Design review of the part built by this model. Coordinates are the model's own, in mm. Round coordinates to 2 decimals unless told otherwise and drop trailing zeros. Order: outer loops, then holes, each group sorted by start corner. A loop starts at its lowest first (then second) coordinate and runs counter-clockwise, first axis right, second up. Notation, with made-up numbers: (63, 89.5) - (78, 89.5) arc R14 cw to (78, 101.5) - close; hole circle Ø11 at (-22, -28). An arc over 180 degrees is marked (long way). Use CSV: the item, a comma, the result in double quotes. Start each with the question number.
from build123d import *

# Parameters (mm, degrees)
SKETCH_1_R      = 2.5
SKETCH_1_R_2    = 11
SKETCH_1_R_3    = 5
SKETCH_1_R_4    = 1.5
EXTRUDE_1_DEPTH = 2


with BuildPart() as part:
    # 草图1 → 凸台-拉伸1 (new body)
    with BuildSketch(Plane.XY):
        with BuildLine():
            Line((-200.597014925, 350), (59.402985075, 350))
            ThreePointArc((59.402985075, 350), (80.61618851, 341.213203436), (89.402985075, 320))
            Line((89.402985075, 320), (89.402985075, -20))
            ThreePointArc((89.402985075, -20), (80.61618851, -41.213203436), (59.402985075, -50))
            Line((59.402985075, -50), (-200.597014925, -50))
            ThreePointArc((-200.597014925, -50), (-221.810218361, -41.213203436), (-230.597014925, -20))
            Line((-230.597014925, -20), (-230.597014925, 320))
            ThreePointArc((-230.597014925, 320), (-221.810218361, 341.213203436), (-200.597014925, 350))
        make_face()
        with Locations((-190.594777504, 260.002592391)):
            Circle(SKETCH_1_R, mode=Mode.SUBTRACT)
        with Locations((49.405222496, 260.002592391)):
            Circle(SKETCH_1_R, mode=Mode.SUBTRACT)
        with Locations((-140.594777504, -9.997407609)):
            Circle(SKETCH_1_R, mode=Mode.SUBTRACT)
        with Locations((-0.594777504, -9.997407609)):
            Circle(SKETCH_1_R, mode=Mode.SUBTRACT)
        with Locations((-110.597014925, 329)):
            Circle(SKETCH_1_R_2, mode=Mode.SUBTRACT)
        with Locations((-30.597014925, 329)):
            Circle(SKETCH_1_R_2, mode=Mode.SUBTRACT)
        with Locations((-190.597014925, 329)):
            Circle(SKETCH_1_R_2, mode=Mode.SUBTRACT)
        with Locations((49.402985075, 329)):
            Circle(SKETCH_1_R_2, mode=Mode.SUBTRACT)
        with Locations((-210.597014925, 35)):
            Circle(SKETCH_1_R_3, mode=Mode.SUBTRACT)
        with Locations((69.402985075, 35)):
            Circle(SKETCH_1_R_3, mode=Mode.SUBTRACT)
        with Locations((-110.599294274, 247.104711047)):
            Circle(SKETCH_1_R_4, mode=Mode.SUBTRACT)
        with Locations((-110.599294274, 153.604711047)):
            Circle(SKETCH_1_R_4, mode=Mode.SUBTRACT)
        with Locations((3.900705726, 153.604711047)):
            Circle(SKETCH_1_R_4, mode=Mode.SUBTRACT)
        with Locations((3.900705726, 247.104711047)):
            Circle(SKETCH_1_R_4, mode=Mode.SUBTRACT)
        with Locations((-200.598097779, 223.669448039)):
            Circle(SKETCH_1_R_4, mode=Mode.SUBTRACT)
        with Locations((-152.398097779, 223.669448039)):
            Circle(SKETCH_1_R_4, mode=Mode.SUBTRACT)
        with Locations((-200.598097779, 175.469448039)):
            Circle(SKETCH_1_R_4, mode=Mode.SUBTRACT)
        with Locations((-152.398097779, 175.469448039)):
            Circle(SKETCH_1_R_4, mode=Mode.SUBTRACT)
        with Locations((-30.597014925, 280)):
            Circle(SKETCH_1_R_3, mode=Mode.SUBTRACT)
        with Locations((-190.594777504, 280)):
            Circle(SKETCH_1_R_3, mode=Mode.SUBTRACT)
        with Locations((-110.599294274, 280)):
            Circle(SKETCH_1_R_3, mode=Mode.SUBTRACT)
        with Locations((49.405222496, 280)):
            Circle(SKETCH_1_R_3, mode=Mode.SUBTRACT)
    extrude(amount=EXTRUDE_1_DEPTH)


solid = part.part
Q1. Take a section at B-B (y = 35). State the section outline as (x, z) points, plus the area to 3 significant figures.
Q2. For L1, parallel to Y at x = 3, z = 0.55; L2, parallel to X at y = 327.5, z = 0.9; L3, parallel to Y at x = -107.5, z = 0.55, list the stretches that pass through material, from the lowest coordinate up. Write a range as [from, to].
Q3. Take a section at C-C (z = 1.25). Give the number of separate pieces and of enclosed holes in the cut face, plus the area to 3 significant figures.
Q4. Take a section at D-D (y = 329). State the section outline as (x, z) points, plus the area to 3 significant figures.
Q5. The part is to be moulded in two halves that separate along Y. For faces 1 (the cylindrical face through (-191.246, 284.957, 0.986)), 2 (the flat face through (-68, 153, 0)), 3 (the cylindrical face through (80.848, -40.979, 0.986)), say which applies: +Y half, -Y half, draft (parallel to the pull), parting line (faces both ways), or undercut.
Q6. Take a section at A-A (y = 280). State the section outline as (x, z) points.
Findings below:
1,outline,"(-230.6, 0) - (-215.6, 0) - (-215.6, 2) - (-230.6, 2) - close; (-205.6, 0) - (64.4, 0) - (64.4, 2) - (-205.6, 2) - close; (74.4, 0) - (89.4, 0) - (89.4, 2) - (74.4, 2) - close"
1,area,"600 mm^2"
2,L1,"y = [-50, 152.41], [154.8, 245.91], [248.3, 350]"
2,L2,"x = [-229.64, -201.49], [-179.7, -121.49], [-99.7, -41.49], [-19.7, 38.51], [60.3, 88.45]"
2,L3,"y = [-50, 276.08], [283.92, 318.44], [339.56, 350]"
3,separate pieces,"1"
3,enclosed holes,"22"
3,area,"125,000 mm^2"
4,outline,"(-229.22, 0) - (-201.6, 0) - (-201.6, 2) - (-229.22, 2) - close; (-179.6, 0) - (-121.6, 0) - (-121.6, 2) - (-179.6, 2) - close; (-99.6, 0) - (-41.6, 0) - (-41.6, 2) - (-99.6, 2) - close; (-19.6, 0) - (38.4, 0) - (38.4, 2) - (-19.6, 2) - close; (60.4, 0) - (88.02, 0) - (88.02, 2) - (60.4, 2) - close"
4,area,"458 mm^2"
5,face 1,"undercut"
5,face 2,"draft"
5,face 3,"-Y half"
6,outline,"(-230.6, 0) - (-195.59, 0) - (-195.59, 2) - (-230.6, 2) - close; (-185.59, 0) - (-115.6, 0) - (-115.6, 2) - (-185.59, 2) - close; (-105.6, 0) - (-35.6, 0) - (-35.6, 2) - (-105.6, 2) - close; (-25.6, 0) - (44.41, 0) - (44.41, 2) - (-25.6, 2) - close; (54.41, 0) - (89.4, 0) - (89.4, 2) - (54.41, 2) - close"
